Design review of the part built by this model. Coordinates are the model's own, in mm. A direction names the side the tool comes from. Give positions to 0.01 mm unless a question says otherwise; leave off trailing zeros. Order: outer loops, then holes, each group sorted by start corner. A loop starts at its lowest first (then second) coordinate and runs counter-clockwise, first axis right, second up. Notation, with made-up numbers: (21, 81.5) -> (53, 81.5) arc R27 ccw to (53, 108.5) -> close; hole circle Ø8 at (-22.5, -10.75). An arc over 180 degrees is marked (long way). Answer in a Markdown table with one row per item. Add a question column.
```python
from build123d import *

# Parameters (mm, degrees)
BOSS_EXTRUDE1_DEPTH = 230
CUT_EXTRUDE1_REACH  = 241.061
SKETCH2_R           = 7.5


with BuildPart() as part:
    # Sketch1 → Boss-Extrude1 (new body)
    with BuildSketch(Plane.XY):
        with BuildLine():
            Line((2.5, -20), (2.5, 30))
            Line((2.5, 30), (-2.5, 30))
            Line((-2.5, 30), (-2.5, -30))
            Line((-2.5, -30), (-2.5, -35))
            Line((-2.5, -35), (57.5, -35))
            Line((57.5, -35), (57.5, -30))
            Line((57.5, -30), (12.5, -30))
            ThreePointArc((12.5, -30), (5.428932188, -27.071067812), (2.5, -20))
        make_face()
    extrude(amount=BOSS_EXTRUDE1_DEPTH)

    # Sketch2 → Cut-Extrude1 (cut, up to next)
    with BuildSketch(Plane(origin=(2.5, 0, 0), x_dir=(0, 0, -1), z_dir=(1, 0, 0)), mode=Mode.PRIVATE) as cut_extrude1_sk1:
        with Locations((-30, 0)):
            Circle(SKETCH2_R)
    cut_extrude1_tool1 = extrude(cut_extrude1_sk1.sketch, amount=-CUT_EXTRUDE1_REACH, mode=Mode.PRIVATE) & part.part
    # Sketch2 → Cut-Extrude1 (cut, up to next)
    with BuildSketch(Plane(origin=(2.5, 0, 0), x_dir=(0, 0, -1), z_dir=(1, 0, 0)), mode=Mode.PRIVATE) as cut_extrude1_sk2:
        with Locations((-180, 0)):
            Circle(SKETCH2_R)
    cut_extrude1_tool2 = extrude(cut_extrude1_sk2.sketch, amount=-CUT_EXTRUDE1_REACH, mode=Mode.PRIVATE) & part.part
    add(cut_extrude1_tool1.solids().sort_by_distance((2.5, 0, 30))[0], mode=Mode.SUBTRACT)
    add(cut_extrude1_tool2.solids().sort_by_distance((2.5, 0, 180))[0], mode=Mode.SUBTRACT)


solid = part.part
```
1) Mouldability with a two-part tool opening along Z and no side actions: class faces 1 (the face through (0.035, 0.33, 37.493)), 2 (the face through (3, -24, 230)), 3 (the face through (0.04, -2.87, 173.07)), 4 (the face through (0, 30, 113)) as +Z half, -Z half, draft (parallel to the pull), parting line (faces both ways), or undercut.
2) Add section B-B, the plane z = 180. Write out the cut boundary in (x, y), and give its area (3 significant figures).
3) Clearance check with flat-ended pins moving along their axes: P1, Ø13.5, axis at x = 37, z = 102, coming from the +Y side; P2, Ø3, axis at x = 6, z = 76, coming from the +Y side. State where each tip first meets the part, or that it passes through.
4) For L1, parallel to Y at x = 0.7, z = 180; L2, parallel to X at y = 13, z = 211; L3, parallel to Y at x = 49, z = 127, list the stretches that pass through material, from the lowest coordinate up.
5) Add section A-A, the plane y = 0. Write out the cut boundary in (x, z), and give its area (3 significant figures).
6) Add section D-D, the plane x = 45. Write out the cut boundary in (y, z).
7) Add section C-C, the plane z = 156. Write out the cut boundary in (x, y), and give its area (3 significant figures).
8) Machinability: for faces 5 (the face through (-2.5, -2, 113)), 6 (the face through (2.5, 5, 113)), which of the approach directions +Z, -Z, +X, -X, +Y, -Y give a long, thin tool a straight path to every point of the face, cutting with its end or side? Answer none if there is none.
Verdict:
| question | item | result |
|---|---|---|
| 1 | face 1 | undercut |
| 1 | face 2 | +Z half |
| 1 | face 3 | undercut |
| 1 | face 4 | draft |
| 2 | outline | (-2.5, -35) -> (57.5, -35) -> (57.5, -30) -> (12.5, -30) arc R10 cw to (2.5, -20) -> (2.5, -7.5) -> (-2.5, -7.5) -> close; (-2.5, 7.5) -> (2.5, 7.5) -> (2.5, 30) -> (-2.5, 30) -> close |
| 2 | area | 546 mm2 |
| 3 | P1 | stops at y = -30 |
| 3 | P2 | stops at y = -26 |
| 4 | L1 | y = -35 to -7.5, 7.5 to 30 |
| 4 | L2 | x = -2.5 to 2.5 |
| 4 | L3 | y = -35 to -30 |
| 5 | outline | (-2.5, 0) -> (2.5, 0) -> (2.5, 22.5) -> (-2.5, 22.5) -> close; (-2.5, 37.5) -> (2.5, 37.5) -> (2.5, 172.5) -> (-2.5, 172.5) -> close; (-2.5, 187.5) -> (2.5, 187.5) -> (2.5, 230) -> (-2.5, 230) -> close |
| 5 | area | 1,000 mm2 |
| 6 | outline | (-35, 0) -> (-30, 0) -> (-30, 230) -> (-35, 230) -> close |
| 7 | outline | (-2.5, -35) -> (57.5, -35) -> (57.5, -30) -> (12.5, -30) arc R10 cw to (2.5, -20) -> (2.5, 30) -> (-2.5, 30) -> close |
| 7 | area | 621 mm2 |
| 8 | face 5 | +Z, -Z, -X, +Y, -Y |
| 8 | face 6 | +Z, -Z, +X, +Y |
